The listing builds one solid part. Answer for the finished solid, in the listing's coordinates (mm). Coordinates: 2 decimals unless noted, no trailing zeros. Order: outer loops, then holes, each group sorted by start corner. A loop starts at its lowest first (then second) coordinate and runs counter-clockwise, first axis right, second up. Notation, with made-up numbers: (22, 68.25) - (42, 68.25) arc R11 cw to (42, 83.25) - close; hole circle Ø7 at (41.5, -28.75). An arc over 180 degrees is marked (long way). One line per item, written item: value. Start each with the question number.
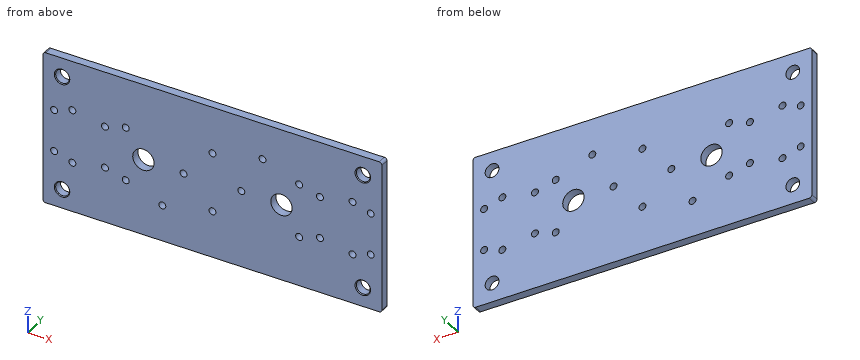
```python
from build123d import *

# Parameters (mm, degrees)
SKETCH1_W                         = 254
SKETCH1_H                         = 114.3
BOSS_EXTRUDE1_DEPTH               = 6.35
M3_CLEARANCE_HOLE1_D              = 5.2
F_3_8_CLEARANCE_HOLE1_D           = 10.31748
F_3_8_CLEARANCE_HOLE1_CSINK_D     = 11.58748
F_3_8_CLEARANCE_HOLE1_CSINK_ANGLE = 90
M3_CLEARANCE_HOLE2_D              = 5.2
FILLET1_R                         = 2
M3_CLEARANCE_HOLE4_D              = 5.2
SKETCH18_R                        = 8
CUT_EXTRUDE1_DEPTH                = 140.411064841


with BuildPart() as part:
    # Sketch1 → Boss-Extrude1 (new body)
    with BuildSketch(Plane(origin=(0, 0, 0), x_dir=(1, 0, 0), z_dir=(0, 1, 0))):
        Rectangle(SKETCH1_W, SKETCH1_H)
    extrude(amount=BOSS_EXTRUDE1_DEPTH)

    # M3 Clearance Hole1 (through all)
    with Locations(Plane(origin=(0, 6.35, 0), x_dir=(1, 0, 0), z_dir=(0, 1, 0))):
        with Locations((-80.5625, -15.621), (-80.5625, 15.621), (-118.6625, -15.621), (-118.6625, 15.621), (118.6625, -15.621), (80.5625, -15.621), (80.5625, 15.621), (118.6625, 15.621)):
            Hole(M3_CLEARANCE_HOLE1_D / 2)

    # 3/8 Clearance Hole1 (through all)
    with Locations(Plane(origin=(0, 0, 0), x_dir=(-1, 0, 0), z_dir=(0, -1, 0))):
        with Locations((-112.7125, 42.8625), (-112.7125, -42.8625), (112.7125, -42.8625), (112.7125, 42.8625)):
            CounterSinkHole(F_3_8_CLEARANCE_HOLE1_D / 2, F_3_8_CLEARANCE_HOLE1_CSINK_D / 2, counter_sink_angle=F_3_8_CLEARANCE_HOLE1_CSINK_ANGLE)

    # M3 Clearance Hole2 (through all)
    with Locations(Plane.XZ):
        with Locations((105, 20), (65, -20), (105, -20), (65, 20), (-65, -20), (-65, 20), (-105, 20), (-105, -20)):
            Hole(M3_CLEARANCE_HOLE2_D / 2)

    # Fillet1
    fillet1_edges = [part.edges().sort_by_distance(p)[0] for p in [
        (-127, 3.175, -57.15),
        (127, 3.175, -57.15),
        (127, 3.175, 57.15),
        (-127, 3.175, 57.15),
    ]]
    fillet(fillet1_edges, radius=FILLET1_R)

    # M3 Clearance Hole4 (through all)
    with Locations(Plane.XZ):
        with Locations((0, -22.1), (-21.65, -0.55), (-37.55, -30.1), (37.55, 30.1), (21.65, 0.55), (0, 22.1)):
            Hole(M3_CLEARANCE_HOLE4_D / 2)

    # Sketch18 → Cut-Extrude1 (cut, through all)
    with BuildSketch(Plane.XZ):
        with Locations(Location((-51.75, 0, 0), (0, 0, 270))):
            Circle(SKETCH18_R)
        with Locations(Location((51.75, 0, 0), (0, 0, 90))):
            Circle(SKETCH18_R)
    extrude(amount=-CUT_EXTRUDE1_DEPTH, mode=Mode.SUBTRACT)


solid = part.part
```
(1) The part is cut by section A-A on x = 65. Determine the outline of the cut face in (y, z), plus the area to 3 significant figures.
(2) The part is cut by section B-B on z = 30.1. Determine the outline of the cut face in (x, y).
(3) The part is cut by section D-D on y = 4.25. Count the separate pieces of the cut face and the enclosed holes in it, plus the area to 3 significant figures.
(4) Consider probe 1 along Z at (x, y) = (65, 3.75); probe 2 along Z at (x, y) = (51.75, 2.5); probe 3 along Z at (x, y) = (-21.65, 2.25). Determine where each line is inside the solid, lowest interval first.
(5) A flat-ended cylindrical pin translates along its axis: pin 1 Ø6 at (x, z) = (112.71, -42.86) entering from -Y. Find the tip coordinate at first contact, or state that the pin passes through.
(6) The part is cut by section C-C on x = -21.65. Determine the outline of the cut face in (y, z), plus the area to 3 significant figures.
Completed:
1. outline: (0, -57.15) - (6.35, -57.15) - (6.35, -22.6) - (0, -22.6) - close; (0, -17.4) - (6.35, -17.4) - (6.35, 17.4) - (0, 17.4) - close; (0, 22.6) - (6.35, 22.6) - (6.35, 57.15) - (0, 57.15) - close
1. area: 660 mm2
2. outline: (-127, 0) - (34.95, 0) - (34.95, 6.35) - (-127, 6.35) - close; (40.15, 0) - (127, 0) - (127, 6.35) - (40.15, 6.35) - close
3. separate pieces: 1
3. enclosed holes: 28
3. area: 27,800 mm2
4. probe 1: z = -57.15 to -22.6, -17.4 to 17.4, 22.6 to 57.15
4. probe 2: z = -57.15 to -8, 8 to 57.15
4. probe 3: z = -57.15 to -3.15, 2.05 to 57.15
5. pin 1: passes through
6. outline: (0, -57.15) - (6.35, -57.15) - (6.35, -3.15) - (0, -3.15) - close; (0, 2.05) - (6.35, 2.05) - (6.35, 57.15) - (0, 57.15) - close
6. area: 693 mm2
